Read the model definition and answer for the solid it produces. Units are mm, in the model's axes. Face numbers are marked on the shaded views. A direction names the side the tool comes from. Coordinates: 2 decimals unless noted, no trailing zeros. Loops run counter-clockwise (first coordinate to the right, second up) from the corner with the lowest first, then second, coordinate; pieces in that order, holes last.
from build123d import *

# Parameters (mm, degrees)
SKETCH_1_R      = 1.6
EXTRUDE_1_DEPTH = 5
FILLET_1_R      = 3


with BuildPart() as part:
    # 草图1 → 凸台-拉伸1 (new body)
    with BuildSketch(Plane.XY):
        Polygon((44.464500341, -26), (44.464500341, 26), (35.964500341, 26), (12, 12), (-12, 12), (-12, -12), (12, -12), (35.964500341, -26), align=None)
        with Locations((40.464500341, -22)):
            Circle(SKETCH_1_R, mode=Mode.SUBTRACT)
        with Locations((40.464500341, 0)):
            Circle(SKETCH_1_R, mode=Mode.SUBTRACT)
        with Locations((40.464500341, 22)):
            Circle(SKETCH_1_R, mode=Mode.SUBTRACT)
        with Locations((-8, -8)):
            Circle(SKETCH_1_R, mode=Mode.SUBTRACT)
        with Locations((-8, 8)):
            Circle(SKETCH_1_R, mode=Mode.SUBTRACT)
        with Locations((8, 8)):
            Circle(SKETCH_1_R, mode=Mode.SUBTRACT)
        with Locations((8, -8)):
            Circle(SKETCH_1_R, mode=Mode.SUBTRACT)
    extrude(amount=EXTRUDE_1_DEPTH)

    # 圆角1
    fillet_1_edges = [part.edges().sort_by_distance(p)[0] for p in [
        (-12, -12, 2.5),
        (-12, 12, 2.5),
        (12, 12, 2.5),
        (35.964500341, 26, 2.5),
        (44.464500341, 26, 2.5),
        (44.464500341, -26, 2.5),
        (35.964500341, -26, 2.5),
        (12, -12, 2.5),
    ]]
    fillet(fillet_1_edges, radius=FILLET_1_R)


solid = part.part
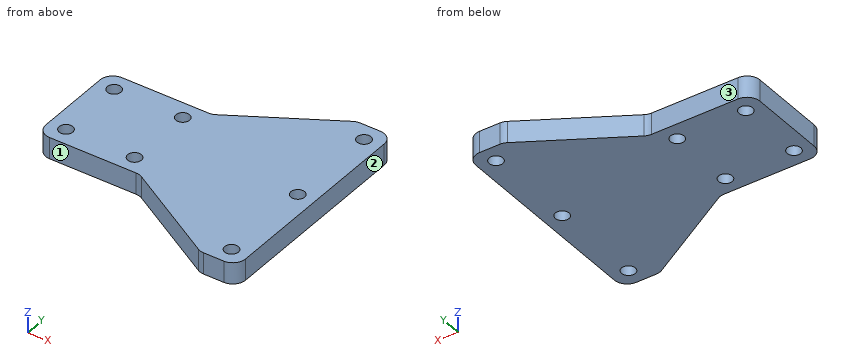
Item 1: Find the intervals of material crossed by line 1 along Y through (x, z) = (8, 2.15); line 2 along Y through (x, z) = (8.5, 1.4); line 3 along Y through (x, z) = (0.5, 1.25), in increasing order.
Numbers:
line 1: y = -12 to -9.6, -6.4 to 6.4, 9.6 to 12
line 2: y = -12 to -9.52, -6.48 to 6.48, 9.52 to 12
line 3: y = -12 to 12
Item 2: A cutting plane is placed at C-C on z = 2.35. Determine the outline of the cut face in (x, y).
Numbers:
outline: (-12, -9) arc R3 ccw to (-9, -12) - (11.19, -12) arc R3 cw to (12.7, -12.41) - (35.26, -25.59) arc R3 ccw to (36.78, -26) - (41.46, -26) arc R3 ccw to (44.46, -23) - (44.46, 23) arc R3 ccw to (41.46, 26) - (36.78, 26) arc R3 ccw to (35.26, 25.59) - (12.7, 12.41) arc R3 cw to (11.19, 12) - (-9, 12) arc R3 ccw to (-12, 9) - close; hole circle Ø3.2 at (-8, -8); hole circle Ø3.2 at (-8, 8); hole circle Ø3.2 at (8, -8); hole circle Ø3.2 at (8, 8); hole circle Ø3.2 at (40.46, -22); hole circle Ø3.2 at (40.46, 0); hole circle Ø3.2 at (40.46, 22)
Item 3: A cutting plane is placed at A-A on x = 8. Determine the outline of the cut face in (y, z).
Numbers:
outline: (-12, 0) - (-9.6, 0) - (-9.6, 5) - (-12, 5) - close; (-6.4, 0) - (6.4, 0) - (6.4, 5) - (-6.4, 5) - close; (9.6, 0) - (12, 0) - (12, 5) - (9.6, 5) - close
Item 4: Which of the six approach directions +Z, -Z, +X, -X, +Y, -Y give full straight-line access (tool end or side, diameter ignored) to the marked faces 1, 2 and 3?
Numbers:
face 1: +Z, -Z, -X, -Y
face 2: +Z, -Z, +X, +Y, -Y
face 3: +Z, -Z, -X, +Y
Item 5: A cutting plane is placed at B-B on y = 0. Determine the outline of the cut face in (x, z).
Numbers:
outline: (-12, 0) - (38.86, 0) - (38.86, 5) - (-12, 5) - close; (42.06, 0) - (44.46, 0) - (44.46, 5) - (42.06, 5) - close
Item 6: Given pin 1 (2 mm diameter, centred on x = 26, z = 1.5, fed in from +Y); pin 2 (2 mm diameter, centred on x = -4.5, z = 1, fed in from +Y); pin 3 (1.5 mm diameter, centred on x = 4.5, z = 1.5, fed in from -Y), each flat-ended and moving along its own axis, determine where each tip first touches the part or whether it passes through.
Numbers:
pin 1: stops at y = 20.76
pin 2: stops at y = 12
pin 3: stops at y = -12
Item 7: A cutting plane is placed at D-D on y = 8. Determine the outline of the cut face in (x, z), then the cut area to 3 significant figures.
Numbers:
outline: (-12, 0) - (-9.6, 0) - (-9.6, 5) - (-12, 5) - close; (-6.4, 0) - (6.4, 0) - (6.4, 5) - (-6.4, 5) - close; (9.6, 0) - (44.46, 0) - (44.46, 5) - (9.6, 5) - close
area: 250 mm2
